Build history of the part. All positions in model axes, mm. Give positions to 0.01 mm unless a question says otherwise; leave off trailing zeros. Order: outer loops, then holes, each group sorted by start corner. A loop starts at its lowest first (then second) coordinate and runs counter-clockwise, first axis right, second up. Notation, with made-up numbers: (21, 41) - (68, 41) arc R20 cw to (68, 58) - close; hole circle Ø11 at (0.5, -28.5). An arc over 180 degrees is marked (long way). Answer in a Markdown table with one row per item.
```python
from build123d import *

# Parameters (mm, degrees)
F0_R     = 1.2446
F1_DEPTH = 11.684
F2_SIZE2 = 1.016
F2_SIZE  = 3.175
F3_R     = 1.5875
F4_DEPTH = 6.35
F5_R     = 2.2479
F6_DEPTH = 4.318
F7_R     = 2.9972
F8_DEPTH = 90.805


with BuildPart() as f1:
    # F0 (on Front) → F1 (new body)
    with BuildSketch(Plane.XZ):
        Circle(F0_R)
    extrude(amount=F1_DEPTH)

    # F2
    f2_edges = [f1.edges().sort_by_distance(p)[0] for p in [
        (-1.2446, 0, 0),
    ]]
    f2_side = f1.faces().sort_by_distance((-1.2446, -5.842, 0))[0]
    chamfer(f2_edges, length=F2_SIZE, length2=F2_SIZE2, reference=f2_side)

    # F3 (on face) → F4 (join)
    with BuildSketch(Plane.XZ.offset(11.684)):
        Circle(F3_R)
    extrude(amount=F4_DEPTH)

    # F5 (on face) → F6 (join)
    with BuildSketch(Plane.XZ.offset(18.034)):
        Circle(F5_R)
    extrude(amount=F6_DEPTH)

    # F7 (on face) → F8 (join)
    with BuildSketch(Plane.XZ.offset(22.352)):
        Circle(F7_R)
    extrude(amount=F8_DEPTH)


solid = f1.part
```
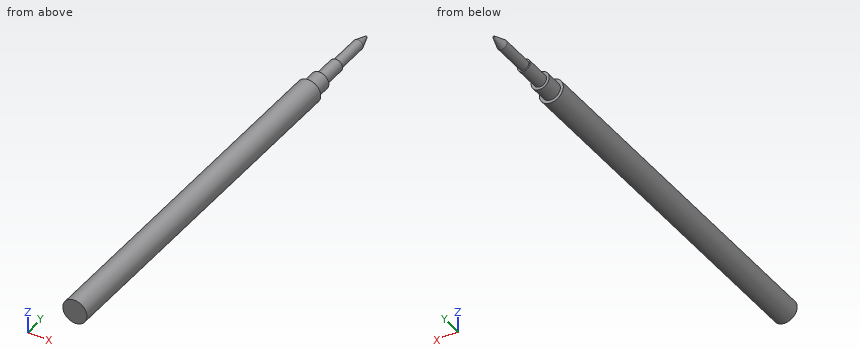
1. Cut at A-A on y = -80. Write the cut outline in (x, z).
Check result:
| item | result |
|---|---|
| outline | circle Ø5.99 at (0, 0) |
2. Probe line 1 (X direction, y = -92, z = -0.2); line 2 (Y direction, x = -0.35, z = 1.25); line 3 (Y direction, x = 1.6, z = -1.9). List the from-to ranges inside material, lowest first.
Check result:
| item | result |
|---|---|
| line 1 | x = -2.99 to 2.99 |
| line 2 | y = -113.16 to -11.68 |
| line 3 | y = -113.16 to -22.35 |
3. Drop flat-ended pins along their axis: P1, Ø3, axis at x = 1, y = -12, coming from the +Z side; P2, Ø1, axis at x = 2.5, y = -91.5, coming from the +Z side. Give the stop position or say it passes through.
Check result:
| item | result |
|---|---|
| P1 | stops at z = 1.59 |
| P2 | stops at z = 2.23 |
4. Cut at B-B on y = -10. Write the cut outline in (x, z), and give its area (3 significant figures).
Check result:
| item | result |
|---|---|
| outline | circle Ø2.49 at (0, 0) |
| area | 4.87 mm² |
